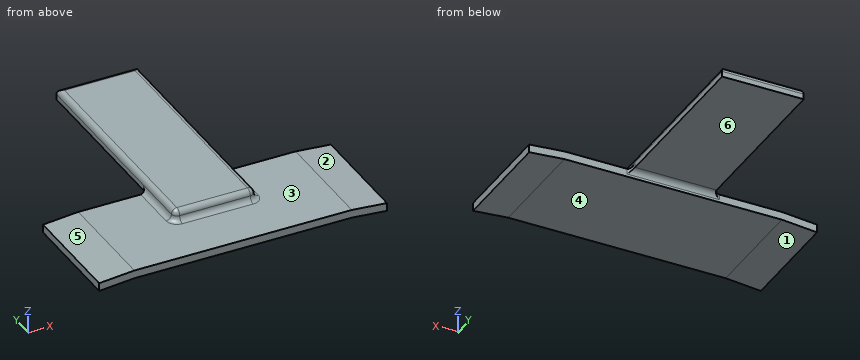
```python
from build123d import *

# Parameters (mm, degrees)
SKETCH1_W           = 101.6
SKETCH1_H           = 50.8
BOSS_EXTRUDE2_DEPTH = 3.8099999999999996
SKETCH2_W           = 50.8
SKETCH2_H           = 16.50999999999999
BOSS_EXTRUDE4_DEPTH = 3.8099999999999996
BOSS_EXTRUDE5_DEPTH = 5.08
FILLET1_R           = 2.54
FILLET18_R          = 2.54
FILLET19_R          = 2.54
FILLET20_R          = 2.54


with BuildPart() as part:
    # Sketch1 → Boss-Extrude2 (new body)
    with BuildSketch(Plane.XY):
        Rectangle(SKETCH1_W, SKETCH1_H)
    extrude(amount=BOSS_EXTRUDE2_DEPTH)

    # Sketch2 → Boss-Extrude4 (add, along a direction that is not the sketch's normal)
    with BuildSketch(Plane(origin=(0.71668285194542, 0, 8.191722482228297), x_dir=(0, 1, 0), z_dir=(-0.08715574274765836, 0, -0.9961946980917455))):
        with Locations((-3.55e-15, 58.52962728319207)):
            Rectangle(SKETCH2_W, SKETCH2_H)
    boss_extrude4 = extrude(amount=BOSS_EXTRUDE4_DEPTH, dir=(0, 0, -1))

    # Mirror1: Boss-Extrude4 across plane
    add(boss_extrude4.mirror(Plane.ZY))

    # Sketch4 → Boss-Extrude5 (add)
    with BuildSketch(Plane.XY.offset(3.8099999999999996)):
        Polygon((-19.05, 0), (19.05, 7e-15), (19.049999999999972, 106.68), (-19.050000000000015, 106.67999999999999), align=None)
    extrude(amount=BOSS_EXTRUDE5_DEPTH)

    # Fillet1
    fillet1_edges = [part.edges().sort_by_distance(p)[0] for p in [
        (-19.05, 12.700000000000003, 3.8099999999999996),
        (0, 3.5e-15, 3.8099999999999996),
        (-19.05, 0, 6.35),
        (19.049999999999997, 12.700000000000001, 3.8099999999999996),
        (19.05, 7e-15, 6.35),
        (-2.132e-14, 106.68, 8.89),
        (-19.050000000000008, 53.339999999999996, 8.89),
        (0, 3.5e-15, 8.89),
        (19.049999999999986, 53.34000000000001, 8.89),
    ]]
    fillet(fillet1_edges, radius=FILLET1_R - 0.0001)  # a hair under: the kernel refuses the full size

    # Fillet18
    fillet18_edges = [part.edges().sort_by_distance(p)[0] for p in [
        (-7.11e-15, 25.399999999999995, 3.8099999999999996),
    ]]
    fillet(fillet18_edges, radius=FILLET18_R)

    # Fillet19
    fillet19_edges = [part.edges().sort_by_distance(p)[0] for p in [
        (19.049999999999994, 25.399999999999995, 3.8099499999999993),
    ]]
    fillet(fillet19_edges, radius=FILLET19_R - 0.0001)  # a hair under: the kernel refuses the full size

    # Fillet20
    fillet20_edges = [part.edges().sort_by_distance(p)[0] for p in [
        (-19.050000000000004, 25.399999999999995, 3.8099499999999997),
    ]]
    fillet(fillet20_edges, radius=FILLET20_R - 0.0001)  # a hair under: the kernel refuses the full size


solid = part.part
```
Here's how the part is built. I have some questions about the finished solid (model axes, mm). Face numbers are marked on the shaded views. A direction names the side the tool comes from. Round coordinates to 2 decimals unless told otherwise and drop trailing zeros. Write each loop counter-clockwise with the first axis right and the second up, starting at its lowest first coordinate (ties: lowest second). Pieces come first, ordered by that corner, then holes.
Q1. Which directions (+Z, -Z, +X, -X, +Y, -Y) give clear straight access to the entire face, cutting with the end or side of a thin tool? Please do the marked faces 4, 5 and 6.
Q2. If we section it at C-C on x = 41: Write out the boundary of the cut face in (y, z), plus the area to 3 significant figures.
Q3. Please list where these lines run through material, in increasing order: probe 1 along Z at (x, y) = (-9, 58); probe 2 along Y at (x, z) = (-23, 2.5); probe 3 along Z at (x, y) = (-40, 0).
Q4. If we section it at D-D on y = 58.5: Write out the boundary of the cut face in (x, z).
Q5. If we mould it in two halves opening along X, with no side actions, what happens to the marked faces 1, 2 and 3? For each: +X half, -X half, draft (parallel to the pull), parting line (faces both ways), or undercut.
Q6. Will these pins go through, and if not, where does the flat tip stop? P1, Ø11.5, axis at x = -2, y = 59.5, coming from the -Z side; P2, Ø10, axis at x = -31, y = 32, coming from the -Z side; P3, Ø4, axis at x = 33.5, z = 0, coming from the +Y side; P4, Ø3, axis at y = 57, z = 5.5, coming from the +X side.
Answer below:
1. face 4: -Z, +Y, -Y
1. face 5: +Z, -X, +Y, -Y
1. face 6: -Z, +X, -X, +Y
2. outline: (-25.4, 0) - (25.4, 0) - (25.4, 3.81) - (-25.4, 3.81) - close
2. area: 194 mm2
3. probe 1: z = 3.81 to 8.89
3. probe 2: y = -25.4 to 25.4
3. probe 3: z = 0 to 3.81
4. outline: (-19.05, 3.81) - (19.05, 3.81) - (19.05, 6.35) arc R2.54 ccw to (16.51, 8.89) - (-16.51, 8.89) arc R2.54 ccw to (-19.05, 6.35) - close
5. face 1: undercut
5. face 2: +X half
5. face 3: draft
6. P1: stops at z = 3.81
6. P2: passes through
6. P3: stops at y = 25.4
6. P4: stops at x = 19.05
